Can you work these out from the model? Positions are in its coordinate system, mm. A direction names the side the tool comes from. Coordinates: 2 decimals unless noted, no trailing zeros. Order: outer loops, then holes, each group sorted by start corner. A loop starts at its lowest first (then second) coordinate and runs counter-clockwise, first axis right, second up. Notation, with made-up numbers: (44.5, 36) -> (94.5, 36) arc R17 ccw to (94.5, 63) -> close; hole circle Ø9 at (21.25, -23.5). An arc over 180 degrees is marked (long way). Return JSON: item names as keys, results as strings. Group by question number.
1) If I drill on probe 1 along Z at (x, y) = (1.1, -12.5); probe 2 along Z at (x, y) = (1.3, 28); probe 3 along Y at (x, z) = (4, 12), over which ranges is the centre line in solid material (lowest first)? Write a range as from..to.
2) If we section it at B-B, the plane y = 15: Please give me the cut outline in (x, z).
3) For faces 4 (the flat face through (3, -22, 40)), 5 (the flat face through (3, -23, -40)), 6 (the flat face through (3, 6.667, 43)), which set-ups out of +Z, -Z, +X, -X, +Y, -Y let a thin tool reach every point of the face, with its end or its side?
4) If we section it at C-C, the plane z = 37: Please give me the cut outline in (x, y), then the cut area to 3 significant figures.
5) For pin 1 (3 mm diameter, centred on x = 3.5, z = -43, fed in from +Y); pin 2 (1.6 mm diameter, centred on x = 4.5, z = 37.5, fed in from +Y); pin 3 (1.8 mm diameter, centred on x = 2, z = -42.5, fed in from -Y), each with a flat end and sliding along its axis, tell me the tip position at first contact or that it passes through.
6) If we section it at D-D, the plane y = -3: Please give me the cut outline in (x, z).
7) If we section it at A-A, the plane z = -30: Please give me the cut outline in (x, y).
8) Thinking about a two-plate mould opening in Y: for faces 1 (the flat face through (3, 0, 32.527)), 2 (the flat face through (3, 28, -7)), 3 (the flat face through (3, 20, -43)), which applies, +Y half, -Y half, draft (parallel to the pull), parting line (faces both ways), or undercut?
from build123d import *

# Parameters (mm, degrees)
F0_R     = 2.5
F0_W     = 35
F0_H     = 2
F1_DEPTH = 5.842


with BuildPart() as f1:
    # F0 (on Right) → F1 (new body)
    with BuildSketch(Plane.YZ):
        Polygon((-25, -35), (-25, -40), (-20, -40), (-20, -45.842), (-6.666667, -45.842), (-6.666667, -40), (6.666667, -40), (6.666667, -45.842), (20, -45.842), (20, -40), (25, -40), (25, -35), (30.842, -35), (30.842, -21), (25, -21), (25, -7), (30.842, -7), (30.842, 7), (25, 7), (25, 21), (30.842, 21), (30.842, 35), (25, 35), (25, 40), (20, 40), (20, 45.842), (6.666667, 45.842), (6.666667, 40), (-6.666667, 40), (-6.666667, 45.842), (-20, 45.842), (-20, 40), (-25, 40), (-25, 35), (-30.842, 35), (-30.842, 21), (-25, 21), (-25, 7), (-30.842, 7), (-30.842, -7), (-25, -7), (-25, -21), (-30.842, -21), (-30.842, -35), align=None)
        with Locations((-3.50444, -30)):
            Circle(F0_R, mode=Mode.SUBTRACT)
        with Locations((3.49556, -30)):
            Circle(F0_R, mode=Mode.SUBTRACT)
        with Locations((0, 30.027077)):
            Rectangle(F0_W, F0_H, mode=Mode.SUBTRACT)
        with Locations((0, 33.527077)):
            Rectangle(F0_W, F0_H, mode=Mode.SUBTRACT)
        with Locations((0, 37.027077)):
            Rectangle(F0_W, F0_H, mode=Mode.SUBTRACT)
    extrude(amount=F1_DEPTH)


solid = f1.part
Result sheet:
{
 "1": {"probe 1": "z = -45.84..29.03, 31.03..32.53, 34.53..36.03, 38.03..45.84", "probe 2": "z = -35..-21, -7..7, 21..35", "probe 3": "y = -25..25"},
 "2": {"outline": "(0, -45.84) -> (5.84, -45.84) -> (5.84, 29.03) -> (0, 29.03) -> close; (0, 31.03) -> (5.84, 31.03) -> (5.84, 32.53) -> (0, 32.53) -> close; (0, 34.53) -> (5.84, 34.53) -> (5.84, 36.03) -> (0, 36.03) -> close; (0, 38.03) -> (5.84, 38.03) -> (5.84, 45.84) -> (0, 45.84) -> close"},
 "3": {"face 4": "+Z, +X, -X, -Y", "face 5": "-Z, +X, -X, -Y", "face 6": "+Z, +X, -X"},
 "4": {"outline": "(0, -25) -> (5.84, -25) -> (5.84, -17.5) -> (0, -17.5) -> close; (0, 17.5) -> (5.84, 17.5) -> (5.84, 25) -> (0, 25) -> close", "area": "87.6 mm2"},
 "5": {"pin 1": "stops at y = 20", "pin 2": "stops at y = 25", "pin 3": "stops at y = -20"},
 "6": {"outline": "(0, -40) -> (5.84, -40) -> (5.84, -32.45) -> (0, -32.45) -> close; (0, -27.55) -> (5.84, -27.55) -> (5.84, 29.03) -> (0, 29.03) -> close; (0, 31.03) -> (5.84, 31.03) -> (5.84, 32.53) -> (0, 32.53) -> close; (0, 34.53) -> (5.84, 34.53) -> (5.84, 36.03) -> (0, 36.03) -> close; (0, 38.03) -> (5.84, 38.03) -> (5.84, 40) -> (0, 40) -> close"},
 "7": {"outline": "(0, -30.84) -> (5.84, -30.84) -> (5.84, -6) -> (0, -6) -> close; (0, -1) -> (5.84, -1) -> (5.84, 1) -> (0, 1) -> close; (0, 6) -> (5.84, 6) -> (5.84, 30.84) -> (0, 30.84) -> close"},
 "8": {"face 1": "undercut", "face 2": "draft", "face 3": "+Y half"}
}
